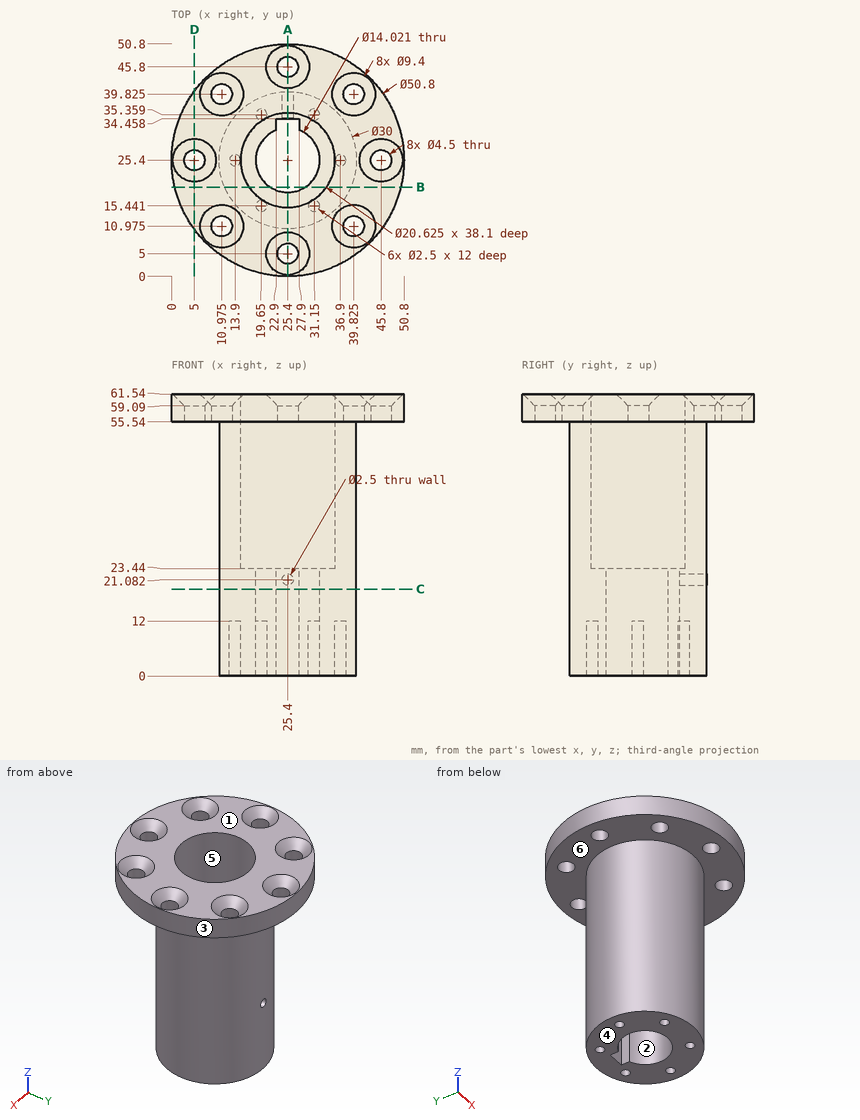
Source: three-view drawing plus pictorial views. Frame: mm from the lowest corner of the part. A direction names the side the tool comes from. Give positions to 0.01 mm unless a question says otherwise; leave off trailing zeros. Loops run counter-clockwise (first coordinate to the right, second up) from the corner with the lowest first, then second, coordinate; pieces in that order, holes last.
1) Contact query for flat-ended pins moving along their axis: pin 1 (10 mm diameter, centred on y = 17.5, z = 23, fed in from -X); pin 2 (2 mm diameter, centred on y = 33, z = 7.5, fed in from -X); pin 3 (1.5 mm diameter, centred on y = 23, z = 8.5, fed in from -X). Output: stop coordinate, or through.
A:
pin 1: stops at x = 10.68
pin 2: stops at x = 11.93
pin 3: stops at x = 10.49
2) Section query B-B on y = 19.5. Return the cut outline in (x, z) (1 decimal), and give its area (3 significant figures).
A:
outline: (0.7, 55.5) - (11.6, 55.5) - (11.6, 0) - (21.6, 0) - (21.6, 23.4) - (16.9, 23.4) - (16.9, 61.5) - (0.7, 61.5) - close; (29.2, 0) - (39.2, 0) - (39.2, 55.5) - (50.1, 55.5) - (50.1, 61.5) - (33.9, 61.5) - (33.9, 23.4) - (29.2, 23.4) - close
area: 1,010 mm2
3) Mould query, pull axis Y, two halves, no side actions, for the marked faces 1, 2 and 3. Classes: released by +Y, released by -Y, zero draft, split by the parting line, or undercut.
A:
face 1: zero draft
face 2: undercut
face 3: split by the parting line
4) Section query C-C on z = 19. Return the cut outline in (x, y).
A:
outline: circle Ø30 at (25.4, 25.4); hole (22.9, 31.95) arc R7.01 ccw (long way) to (27.9, 31.95) - (27.9, 34.46) - (22.9, 34.46) - close
5) Reachability of the marked faces 4, 5 and 6 from +Z, -Z, +X, -X, +Y, -Y: full face, straight path, thin tool, end or side. Return the list, or none.
A:
face 4: -Z, +X, -X, +Y, -Y
face 5: +Z
face 6: -Z
6) Section query A-A on x = 25.4. Count the separate pieces of the cut face and the enclosed holes in it.
A:
separate pieces: 5
enclosed holes: 0
7) Line query: L1, parallel to Y at x = 25.4, z = 40; L2, parallel to Y at x = 23.5, z = 58.5 (1 decimal); L3, parallel to Y at x = 25.4, z = 10.25. Output: solid intervals per line, ascending.
A:
L1: y = 10.4 to 15.09, 35.71 to 40.4
L2: y = 0.1 to 3.8, 6.2 to 15.3, 35.5 to 44.6, 47 to 50.7
L3: y = 10.4 to 18.39, 34.46 to 40.4
8) Section query D-D on x = 5. Return the cut outline in (y, z), and give its area (3 significant figures).
A:
outline: (10.27, 55.54) - (23.15, 55.54) - (23.15, 59.09) - (20.7, 61.54) - (10.27, 61.54) - close; (27.65, 55.54) - (40.53, 55.54) - (40.53, 61.54) - (30.1, 61.54) - (27.65, 59.09) - close
area: 149 mm2
